Part model, mm, in its own coordinate system. A direction names the side the tool comes from. Give positions to 0.01 mm unless a question says otherwise; leave off trailing zeros. Write each loop counter-clockwise with the first axis right and the second up, starting at its lowest first coordinate (ties: lowest second). Pieces come first, ordered by that corner, then holes. Notation, with made-up numbers: (20, -40) - (36, -40) arc R14 ccw to (36, -36) - close; hole circle Ø7 at (-30, 46). An arc over 180 degrees is marked (long way). Answer in a Markdown table with one row per item. Add a question column.
1. Band-saw the part on D-D on z = -16. Write the cut outline in (x, y), plus the area to 3 significant figures.
2. Band-saw the part on A-A on x = 0. Write the cut outline in (y, z).
3. Band-saw the part on C-C on x = -31. Write the cut outline in (y, z), plus the area to 3 significant figures.
4. Which spindle directions (+Z, -Z, +X, -X, +Y, -Y) get a long thin tool onto all of the face, cutting with end or side? Do faces 1 (the cylindrical face through (-39, 0, 38)), 2 (the flat face through (-35, 0, 38)). Say none if no direction does.
5. Probe line 1 along Y through (x, z) = (0, -7); line 2 along Y through (x, z) = (2, 14); line 3 along X through (y, z) = (1.5, -21). List the from-to ranges inside material, lowest first.
6. Drop flat-ended pins along their axis: pin 1 Ø2.5 at (x, z) = (-4, 36.5) entering from +Y; pin 2 Ø5.5 at (y, z) = (-15, 37) entering from -X; pin 3 Ø5 at (x, y) = (-15, 28.5) entering from +Z; pin 4 Ø2.5 at (x, z) = (-3, 37.5) entering from -Y. Give the stop position or say it passes through.
7. Pull direction X, two halves, no side cores. Call faces 3 (the cylindrical face through (-39, 38, 0)), 4 (the flat face through (0, 35, 38)), 5 (the flat face through (0, -40, 0)): released by +X, released by -X, zero draft, split by the parting line, or undercut.
```python
from build123d import *

# Parameters (mm, degrees)
F0_W     = 80
F0_H     = 80
F1_DEPTH = 40
F2_R     = 5
F3_R     = 15
F4_DEPTH = 80.001
F5_R     = 5
F6_DEPTH = 5


with BuildPart() as f1:
    # F0 (on Top) → F1 (new body, symmetric)
    with BuildSketch(Plane.XY):
        Rectangle(F0_W, F0_H)
    extrude(amount=F1_DEPTH, both=True)

    # F2
    f2_edges = [f1.edges().sort_by_distance(p)[0] for p in [
        (0, 40, 40),
        (-40, 0, 40),
        (0, -40, 40),
        (40, 0, 40),
        (-40, 40, 0),
        (0, 40, -40),
        (-40, 0, -40),
        (-40, -40, 0),
        (40, -40, 0),
        (40, 0, -40),
        (40, 40, 0),
        (0, -40, -40),
    ]]
    fillet(f2_edges, radius=F2_R)

    # F3 (on face) → F4 (cut, through all)
    with BuildSketch(Plane.XY.offset(40)):
        Circle(F3_R)
    extrude(amount=-F4_DEPTH, mode=Mode.SUBTRACT)

    # F5
    f5_edges = [f1.edges().sort_by_distance(p)[0] for p in [
        (-15, 0, -40),
    ]]
    fillet(f5_edges, radius=F5_R)

    # F6 (cut): a face of the model
    f6_faces = [f1.faces().sort_by_distance(p)[0] for p in [
        (0, 34.0100505063, 40),
    ]]
    extrude(f6_faces, amount=-F6_DEPTH, mode=Mode.SUBTRACT)


solid = f1.part
```
Values:
| question | item | result |
|---|---|---|
| 1 | outline | (-40, -35) arc R5 ccw to (-35, -40) - (35, -40) arc R5 ccw to (40, -35) - (40, 35) arc R5 ccw to (35, 40) - (-35, 40) arc R5 ccw to (-40, 35) - close; hole circle Ø30 at (0, 0) |
| 1 | area | 5,670 mm² |
| 2 | outline | (-40, -35) arc R5 ccw to (-35, -40) - (-20, -40) arc R5 ccw to (-15, -35) - (-15, 35) - (-35, 35) - (-35, 40) arc R5 ccw to (-40, 35) - close; (15, -35) arc R5 ccw to (20, -40) - (35, -40) arc R5 ccw to (40, -35) - (40, 35) arc R5 ccw to (35, 40) - (35, 35) - (15, 35) - close |
| 3 | outline | (-40, -35) arc R5 ccw to (-35, -40) - (35, -40) arc R5 ccw to (40, -35) - (40, 35) arc R5 ccw to (35, 40) - (35, 35) - (-35, 35) - (-35, 40) arc R5 ccw to (-40, 35) - close |
| 3 | area | 6,030 mm² |
| 4 | face 1 | +Z, -X, +Y, -Y |
| 4 | face 2 | +Z |
| 5 | line 1 | y = -40 to -15, 15 to 40 |
| 5 | line 2 | y = -40 to -14.87, 14.87 to 40 |
| 5 | line 3 | x = -40 to -14.92, 14.92 to 40 |
| 6 | pin 1 | stops at y = 39.99 |
| 6 | pin 2 | stops at x = -40 |
| 6 | pin 3 | stops at z = 35 |
| 6 | pin 4 | stops at y = -39.84 |
| 7 | face 3 | released by -X |
| 7 | face 4 | undercut |
| 7 | face 5 | zero draft |
